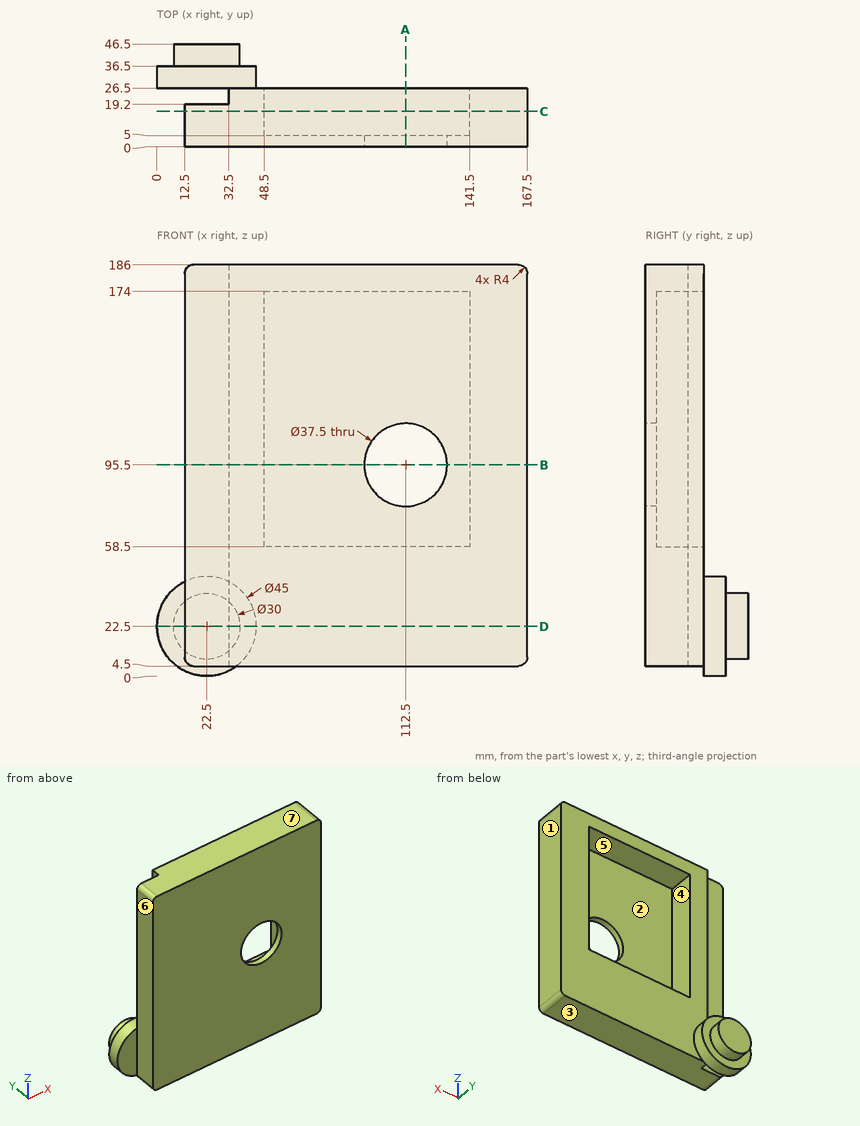
Part print with two shaded views. Sizes in mm from the minimum x, y, z corner. A direction names the side the tool comes from. Round coordinates to 2 decimals unless told otherwise and drop trailing zeros. Order: outer loops, then holes, each group sorted by start corner. A loop starts at its lowest first (then second) coordinate and runs counter-clockwise, first axis right, second up. Notation, with made-up numbers: (16.25, 63) - (22.25, 63) arc R18 ccw to (22.25, 68) - close; hole circle Ø2 at (87, 7). An arc over 180 degrees is marked (long way). Answer in a Markdown table with one row per item. Add a question column.
(1) Band-saw the part on D-D on z = 22.5. List the corners of the cut face in (x, y).
(2) 3-axis set-ups, long thin cutter, end or side, ignore diameter. For the marked faces 5, 6 and 7: which of +Z, -Z, +X, -X, +Y, -Y reach the whole face in a straight line?
(3) Band-saw the part on B-B on z = 95.5. List the corners of the cut face in (x, y).
(4) Drop flat-ended pins along their axis: pin 1 Ø1 at (y, z) = (15, 86.5) entering from -X; pin 2 Ø5 at (x, z) = (119.5, 109.5) entering from -Y; pin 3 Ø3.5 at (y, z) = (22.5, 67) entering from -X; pin 4 Ø5 at (x, y) = (88, 22) entering from -Z. Give the stop position or say it passes through.
(5) Mould opens along X. For the marked faces 1, 2, 3 and 4 say: +X half, -X half, draft (parallel to the pull), parting line (faces both ways), or undercut.
(6) Band-saw the part on A-A on x = 112.5. List the corners of the cut face in (y, z), and give its area (3 significant figures).
(7) Band-saw the part on C-C on y = 16. List the corners of the cut face in (x, z), and give its area (3 significant figures).
(8) Probe L1, parallel to X at y = 6.5, z = 169; L2, parallel to Z at x = 112, y = 1; L3, parallel to Z at x = 61, y = 19.5. List the from-to ranges inside material, lowest first. Write a range as [from, to].
Data:
| question | item | result |
|---|---|---|
| 1 | outline | (0, 26.5) - (32.5, 26.5) - (32.5, 19.2) - (12.5, 19.2) - (12.5, 0) - (167.5, 0) - (167.5, 26.5) - (45, 26.5) - (45, 36.5) - (37.5, 36.5) - (37.5, 46.5) - (7.5, 46.5) - (7.5, 36.5) - (0, 36.5) - close |
| 2 | face 5 | +Y |
| 2 | face 6 | +Z, -Z, -X, -Y |
| 2 | face 7 | +Z, +X, -X, +Y, -Y |
| 3 | outline | (12.5, 0) - (93.75, 0) - (93.75, 5) - (48.5, 5) - (48.5, 26.5) - (32.5, 26.5) - (32.5, 19.2) - (12.5, 19.2) - close; (131.25, 0) - (167.5, 0) - (167.5, 26.5) - (141.5, 26.5) - (141.5, 5) - (131.25, 5) - close |
| 4 | pin 1 | stops at x = 12.5 |
| 4 | pin 2 | passes through |
| 4 | pin 3 | stops at x = 32.5 |
| 4 | pin 4 | stops at z = 4.5 |
| 5 | face 1 | +X half |
| 5 | face 2 | undercut |
| 5 | face 3 | draft |
| 5 | face 4 | undercut |
| 6 | outline | (0, 4.5) - (26.5, 4.5) - (26.5, 58.5) - (5, 58.5) - (5, 76.75) - (0, 76.75) - close; (0, 114.25) - (5, 114.25) - (5, 174) - (26.5, 174) - (26.5, 186) - (0, 186) - close |
| 6 | area | 2,140 mm^2 |
| 7 | outline | (12.5, 8.5) arc R4 ccw to (16.5, 4.5) - (163.5, 4.5) arc R4 ccw to (167.5, 8.5) - (167.5, 182) arc R4 ccw to (163.5, 186) - (16.5, 186) arc R4 ccw to (12.5, 182) - close; hole (48.5, 58.5) - (141.5, 58.5) - (141.5, 174) - (48.5, 174) - close |
| 7 | area | 17,400 mm^2 |
| 8 | L1 | x = [12.5, 48.5], [141.5, 167.5] |
| 8 | L2 | z = [4.5, 76.76], [114.24, 186] |
| 8 | L3 | z = [4.5, 58.5], [174, 186] |
